from build123d import *

# Parameters (mm, degrees)
F0_R     = 1.25
F1_DEPTH = 6
F2_R     = 1.25
F3_DEPTH = 3
F4_SIZE  = 2.99999
F5_R     = 3.175
F6_DEPTH = 3
F7_R     = 3.675
F7_R_2   = 3.175
F8_DEPTH = 6


# Not quite as in the source:
# - a fillet or chamfer is up to 0.001 mm smaller than in the source, because OpenCascade refuses the exact size


with BuildPart() as f1:
    # F0 (on Front) → F1 (new body)
    with BuildSketch(Plane.XZ):
        with BuildLine():
            Line((22.9103805721, 41.8708454072), (-24.0896194279, 41.8708454072))
            ThreePointArc((-24.0896194279, 41.8708454072), (-26.9180465527, 40.699272532), (-28.0896194279, 37.8708454072))
            Line((-28.0896194279, 37.8708454072), (-28.0896194279, -34.1291545928))
            ThreePointArc((-28.0896194279, -34.1291545928), (-26.9180465527, -36.9575817175), (-24.0896194279, -38.1291545928))
            Line((-24.0896194279, -38.1291545928), (22.9103805721, -38.1291545928))
            ThreePointArc((22.9103805721, -38.1291545928), (25.7388076968, -36.9575817175), (26.9103805721, -34.1291545928))
            Line((26.9103805721, -34.1291545928), (26.9103805721, 37.8708454072))
            ThreePointArc((26.9103805721, 37.8708454072), (25.7388076968, 40.699272532), (22.9103805721, 41.8708454072))
        make_face()
        with Locations((-21.5896194279, -32.1291545928)):
            Circle(F0_R, mode=Mode.SUBTRACT)
        with Locations((20.4103805721, -32.1291545928)):
            Circle(F0_R, mode=Mode.SUBTRACT)
        Polygon((5.7612335332, 1.8708454072), (2.5858070526, -3.6291545928), (-3.7650459085, -3.6291545928), (-6.940472389, 1.8708454072), (-3.7650459085, 7.3708454072), (2.5858070526, 7.3708454072), align=None, mode=Mode.SUBTRACT)
        with Locations((-21.5896194279, 35.8708454072)):
            Circle(F0_R, mode=Mode.SUBTRACT)
        with Locations((20.4103805721, 35.8708454072)):
            Circle(F0_R, mode=Mode.SUBTRACT)
    extrude(amount=F1_DEPTH)

    # F2 (on face) → F3 (cut)
    with BuildSketch(Plane(origin=(0, 0, 0), x_dir=(-1, 0, 0), z_dir=(0, 1, 0))):
        with BuildLine():
            ThreePointArc((28.0896194279, 37.8708454072), (26.9180465527, 40.699272532), (24.0896194279, 41.8708454072))
            Line((24.0896194279, 41.8708454072), (-22.9103805721, 41.8708454072))
            ThreePointArc((-22.9103805721, 41.8708454072), (-25.7388076968, 40.699272532), (-26.9103805721, 37.8708454072))
            Line((-26.9103805721, 37.8708454072), (-26.9103805721, -34.1291545928))
            ThreePointArc((-26.9103805721, -34.1291545928), (-25.7388076968, -36.9575817175), (-22.9103805721, -38.1291545928))
            Line((-22.9103805721, -38.1291545928), (24.0896194279, -38.1291545928))
            ThreePointArc((24.0896194279, -38.1291545928), (26.9180465527, -36.9575817175), (28.0896194279, -34.1291545928))
            Line((28.0896194279, -34.1291545928), (28.0896194279, 37.8708454072))
        make_face()
        with Locations((-20.4103805721, -32.1291545928)):
            Circle(F2_R, mode=Mode.SUBTRACT)
        with Locations((21.5896194279, -32.1291545928)):
            Circle(F2_R, mode=Mode.SUBTRACT)
        Polygon((13.2913253501, 1.8708454072), (6.940472389, -9.1291545928), (-5.7612335332, -9.1291545928), (-12.1120864943, 1.8708454072), (-5.7612335332, 12.8708454072), (6.940472389, 12.8708454072), align=None, mode=Mode.SUBTRACT)
        with Locations((-20.4103805721, 35.8708454072)):
            Circle(F2_R, mode=Mode.SUBTRACT)
        with Locations((21.5896194279, 35.8708454072)):
            Circle(F2_R, mode=Mode.SUBTRACT)
    extrude(amount=-F3_DEPTH, mode=Mode.SUBTRACT)

    # F4 (size 3 in the source; OpenCascade refuses exactly that, so slightly less here)
    f4_edges = [f1.edges().sort_by_distance(p)[0] for p in [
        (8.93666, -3, 7.370845),
        (8.93666, -3, -3.629155),
        (-0.589619, -3, -9.129155),
        (-10.115899, -3, -3.629155),
        (-10.115899, -3, 7.370845),
        (-0.589619, -3, 12.870845),
    ]]
    chamfer(f4_edges, length=F4_SIZE)

    # F5 (on face) → F6 (join)
    with BuildSketch(Plane(origin=(0, 0, 0), x_dir=(-1, 0, 0), z_dir=(0, 1, 0))):
        Polygon((6.940472389, -9.1291545928), (13.2913253501, 1.8708454072), (6.940472389, 12.8708454072), (-5.7612335332, 12.8708454072), (-12.1120864943, 1.8708454072), (-5.7612335332, -9.1291545928), align=None)
        Polygon((3.7650459085, -3.6291545928), (-2.5858070526, -3.6291545928), (-5.7612335332, 1.8708454072), (-2.5858070526, 7.3708454072), (3.7650459085, 7.3708454072), (6.940472389, 1.8708454072), align=None, mode=Mode.SUBTRACT)
        Polygon((-5.7612335332, 1.8708454072), (-2.5858070526, -3.6291545928), (3.7650459085, -3.6291545928), (6.940472389, 1.8708454072), (3.7650459085, 7.3708454072), (-2.5858070526, 7.3708454072), align=None)
        with Locations((0.5896194279, 1.8708454072)):
            Circle(F5_R, mode=Mode.SUBTRACT)
    extrude(amount=F6_DEPTH)

    # F7 (on face) → F8 (join, through all)
    with BuildSketch(Plane.XZ):
        with Locations((-0.5896194279, 1.8708454072)):
            Circle(F7_R)
        with Locations((-0.5896194279, 1.8708454072)):
            Circle(F7_R_2, mode=Mode.SUBTRACT)
    extrude(amount=F8_DEPTH)


solid = f1.part
Can you work these out from the model? Positions are in its coordinate system, mm. A direction names the side the tool comes from. Coordinates: 2 decimals unless noted, no trailing zeros. Write each loop counter-clockwise with the first axis right and the second up, starting at its lowest first coordinate (ties: lowest second). Pieces come first, ordered by that corner, then holes. Notation, with made-up numbers: (-18.5, -29.75) -> (15.5, -29.75) arc R33 cw to (15.5, -0.75) -> close; hole circle Ø9 at (59, -22). An arc over 180 degrees is marked (long way). Write each question's results on one line, items separated by ' | '. Start each with the question number.
Q1. Imagine slicing it at C-C (x = 9). Write out the boundary of the cut face in (y, z).
Q2. Imagine slicing it at D-D (x = -19). Write out the boundary of the cut face in (y, z), then the cut area to 3 significant figures.
Q3. On a 3-axis mill with a long thin cutter (end or side, diameter ignored), from which of +Z, -Z, +X, -X, +Y, -Y can I reach the whole of each face in a straight line? I mean faces 5 (the face through (25.77, -4.48, 40.67)), 6 (the face through (-1, -3, -3.629)), 7 (the face through (8.89, 1.48, 7.45)), 8 (the face through (-10.16, 1.479, 7.294)), 9 (the face through (-1, 1, 12.871)). Say none if no direction works.
Q4. I'm going to push flat-ended pins straight in: pin 1 (0.9 mm diameter, centred on x = -1.5, y = 1.5, fed in from -Z); pin 2 (3 mm diameter, centred on x = 20.41, z = -32.13, fed in from +Y); pin 3 (3.5 mm diameter, centred on x = 0.5, y = 1.5, fed in from +Z). Where does each tip first touch, or does it pass through?
Q5. Imagine slicing it at B-B (z = -7.5). Write out the boundary of the cut face in (x, y).
Q6. Imagine slicing it at A-A (x = 0). Write out the boundary of the cut face in (y, z).
Q7. We'd pull the mould along X, two halves only. Please class faces 1 (the face through (8.981, 1.479, -3.552)), 2 (the face through (-1, 1, -9.129)), 3 (the face through (-5.375, -2.958, 4.582)), 4 (the face through (-11.49, -1.52, -4.29)): +X half, -X half, draft (parallel to the pull), parting line (faces both ways), or undercut.
Q8. If I drill on probe 1 along Z at (x, y) = (-2.5, -1); probe 2 along X at (y, z) = (-4, -1); probe 3 along Y at (x, z) = (-19, 5), over which ranges is the centre line in solid material (lowest first)?
Taken from the geometry:
1) outline: (-6, -38.13) -> (-3, -38.13) -> (-3, -9.52) -> (0, -3.52) -> (3, -3.52) -> (3, 7.26) -> (0, 7.26) -> (-3, 13.26) -> (-3, 41.87) -> (-6, 41.87) -> close
2) outline: (-6, -38.13) -> (-3, -38.13) -> (-3, 41.87) -> (-6, 41.87) -> close | area: 240 mm^2
3) face 5: +Z, +X, +Y, -Y | face 6: -Y | face 7: +Z, +X, +Y | face 8: +Z, -X, +Y | face 9: +Z, +X, -X, +Y
4) pin 1: stops at z = -9.13 | pin 2: stops at y = -3 | pin 3: stops at z = 13.12
5) outline: (-28.09, -6) -> (26.91, -6) -> (26.91, -3) -> (10.17, -3) -> (6.7, 0) -> (6.7, 3) -> (-7.88, 3) -> (-7.88, 0) -> (-11.35, -3) -> (-28.09, -3) -> close
6) outline: (-6, -38.13) -> (-3, -38.13) -> (-3, -12.13) -> (0, -9.13) -> (3, -9.13) -> (3, -1.25) -> (-6, -1.25) -> (-6, -1.76) -> (0, -1.76) -> (0, -3.63) -> (-6, -3.63) -> close; (-6, 4.99) -> (3, 4.99) -> (3, 12.87) -> (0, 12.87) -> (-3, 15.87) -> (-3, 41.87) -> (-6, 41.87) -> (-6, 7.37) -> (0, 7.37) -> (0, 5.5) -> (-6, 5.5) -> close
7) face 1: +X half | face 2: draft | face 3: undercut | face 4: -X half
8) probe 1: z = -10.13 to -3.63, -1.27 to -0.67, 4.41 to 5.01, 7.37 to 13.87 | probe 2: x = -28.09 to -5.28, -2.88 to -1.95, 0.77 to 1.7, 4.1 to 26.91 | probe 3: y = -6 to -3
